For this review, take the finished solid that the model builds, in its own axes (mm). A direction names the side the tool comes from. Coordinates: 2 decimals unless noted, no trailing zeros. Write each loop counter-clockwise with the first axis right and the second up, starting at its lowest first coordinate (ties: lowest second). Pieces come first, ordered by that corner, then holes. Notation, with made-up numbers: (-4.75, 45.25) - (-0.75, 45.25) arc R16 cw to (-0.75, 50.25) - close; hole circle Ø5 at (4.25, -17). An arc over 180 degrees is marked (long way). Use one line per item in the form item = value. Start each with the question number.
1) We need section B-B (x = 0). Give the boundary of the cut face in (y, z), plus the area to 3 significant figures.
2) We need section D-D (y = 5). Count the separate pieces of the cut face and the enclosed holes in it, plus the area to 3 significant figures.
3) We need section A-A (z = 16.5). Give the boundary of the cut face in (x, y).
4) We need section C-C (y = -19.25). Give the boundary of the cut face in (x, z).
5) Mouldability with a two-part tool opening along Z and no side actions: class faces 5 (the flat face through (-12, 0, 1)), 6 (the flat face through (12, 0, 3)), 7 (the cylindrical face through (54.01, 5.09, 25.05)), 8 (the cylindrical face through (24.854, 16.483, 1.986)) as pulls with the +Z half, pulls with the -Z half, needs draft (parallel to the pull), parting line crosses it, or undercut.
6) Tool access review of faces 1 (the flat face through (-13.752, -7.982, 1.986)), 2 (the flat face through (53, 5, 16)), 3 (the cylindrical face through (54.1, 4.86, 1.86)), 4 (the flat face through (-54, -5, 14)): name each direction out of +Z, -Z, +X, -X, +Y, -Y from which nothing blocks a thin tool from reaching the whole face with its end or side.
7) Insertion check: P1, Ø6.5, axis at x = -25.11, y = 14.5, coming from the +Z side; P2, Ø3.5, axis at x = -53, z = 12, coming from the +Y side; P3, Ø1.5, axis at x = -54, z = 18, coming from the -Y side. Each pin has a flat end and moves straight along its axis. Give the tip position at first contact, or say it passes through.
8) For L1, parallel to Y at x = 0, z = 2.2; L2, parallel to X at y = 13, z = 19.25; L3, parallel to Y at x = 53.85, z = 23, list the stretches that pass through material, from the lowest coordinate up. Write a range as from..to.
```python
from build123d import *

# Parameters (mm, degrees)
SKETCH_1_R                  = 33
SKETCH_1_R_2                = 11.05
SKETCH_1_R_3                = 4.05
SKETCH_1_R_4                = 2
EXTRUDE_1_DEPTH             = 3
EXTRUDE_2_DEPTH             = 3
SHEET_METAL_1_OUTLINE_R     = 2
SHEET_METAL_1_OUTLINE_R_2   = 4.05
SHEET_METAL_1_OUTLINE_R_3   = 11.05
SHEET_METAL_1_DEPTH         = 1
SM_EDGE_FLANGE_1_DEPTH      = 20
SM_EDGE_FLANGE_1_BEND_DEPTH = 20
SKETCH_13_R                 = 2.05
CUT_EXTRUDE_1_DEPTH         = 118.974573532


# Read off the part's stored shape, not the designer's step: 转换实体1
# Sheet-metal steps are written as plain solids
with BuildPart() as part:
    # Sketch 1 → 凸台-拉伸1 (new body)
    with BuildSketch(Plane.XY):
        Circle(SKETCH_1_R)
        Circle(SKETCH_1_R_2, mode=Mode.SUBTRACT)
        with Locations((0, -19.25)):
            Circle(SKETCH_1_R_3, mode=Mode.SUBTRACT)
        with Locations((25.11473671, 14.5)):
            Circle(SKETCH_1_R_4, mode=Mode.SUBTRACT)
        with Locations((0, -29)):
            Circle(SKETCH_1_R_4, mode=Mode.SUBTRACT)
        with Locations((-25.11473671, 14.5)):
            Circle(SKETCH_1_R_4, mode=Mode.SUBTRACT)
        with BuildLine():
            Line((-19.57313602, -8.29833395), (-16.97313602, -12.80166605))
            ThreePointArc((-16.97313602, -12.80166605), (-16.487370933, -13.174406711), (-15.880315697, -13.094486373))
            Line((-15.880315697, -13.094486373), (-12.762624243, -11.294486373))
            ThreePointArc((-12.762624243, -11.294486373), (-12.389883582, -10.808721286), (-12.46980392, -10.20166605))
            Line((-12.46980392, -10.20166605), (-15.06980392, -5.69833395))
            ThreePointArc((-15.06980392, -5.69833395), (-15.555569007, -5.325593289), (-16.162624243, -5.405513627))
            Line((-16.162624243, -5.405513627), (-19.280315697, -7.205513627))
            ThreePointArc((-19.280315697, -7.205513627), (-19.653056358, -7.691278714), (-19.57313602, -8.29833395))
        make_face(mode=Mode.SUBTRACT)
    extrude(amount=EXTRUDE_1_DEPTH)

    # 草图3 → 凸台-拉伸2 (add)
    with BuildSketch(Plane.XY):
        with BuildLine():
            ThreePointArc((-18.301945503, -27.459766765), (-32.813072233, 3.507462139), (-12.084283208, 30.707818212))
            Line((-12.084283208, 30.707818212), (-52, 15))
            Line((-52, 15), (-52, -5))
            Line((-52, -5), (-18.301945503, -27.459766765))
        make_face()
        with BuildLine():
            ThreePointArc((18.301945503, -27.459766765), (32.813072233, 3.507462139), (12.084283208, 30.707818212))
            Line((12.084283208, 30.707818212), (52, 15))
            Line((52, 15), (52, -5))
            Line((52, -5), (18.301945503, -27.459766765))
        make_face()
    extrude(amount=EXTRUDE_2_DEPTH)

    # Sheet Metal 1 outline → Sheet Metal 1 (cut)
    with BuildSketch(Plane.XY):
        with BuildLine():
            ThreePointArc((-18.301945503, -27.459766765), (0, -33), (18.301945503, -27.459766765))
            Line((18.301945503, -27.459766765), (52, -5))
            Line((52, -5), (52, 15))
            Line((52, 15), (12.084283208, 30.707818212))
            ThreePointArc((12.084283208, 30.707818212), (0, 33), (-12.084283208, 30.707818212))
            Line((-12.084283208, 30.707818212), (-52, 15))
            Line((-52, 15), (-52, -5))
            Line((-52, -5), (-18.301945503, -27.459766765))
        make_face()
        with BuildLine():
            Line((-16.97313602, -12.80166605), (-19.57313602, -8.29833395))
            ThreePointArc((-19.57313602, -8.29833395), (-19.653056358, -7.691278714), (-19.280315697, -7.205513627))
            Line((-19.280315697, -7.205513627), (-16.162624243, -5.405513627))
            ThreePointArc((-16.162624243, -5.405513627), (-15.555569007, -5.325593289), (-15.06980392, -5.69833395))
            Line((-15.06980392, -5.69833395), (-12.46980392, -10.20166605))
            ThreePointArc((-12.46980392, -10.20166605), (-12.389883582, -10.808721286), (-12.762624243, -11.294486373))
            Line((-12.762624243, -11.294486373), (-15.880315697, -13.094486373))
            ThreePointArc((-15.880315697, -13.094486373), (-16.487370933, -13.174406711), (-16.97313602, -12.80166605))
        make_face(mode=Mode.SUBTRACT)
        with Locations((0, -29)):
            Circle(SHEET_METAL_1_OUTLINE_R, mode=Mode.SUBTRACT)
        with Locations((0, -19.25)):
            Circle(SHEET_METAL_1_OUTLINE_R_2, mode=Mode.SUBTRACT)
        with Locations((-25.11473671, 14.5)):
            Circle(SHEET_METAL_1_OUTLINE_R, mode=Mode.SUBTRACT)
        Circle(SHEET_METAL_1_OUTLINE_R_3, mode=Mode.SUBTRACT)
        with Locations((25.11473671, 14.5)):
            Circle(SHEET_METAL_1_OUTLINE_R, mode=Mode.SUBTRACT)
    extrude(amount=SHEET_METAL_1_DEPTH, mode=Mode.SUBTRACT)

    # 边线-法兰1 section (across the edge) → 边线-法兰1 (add)
    with BuildSketch(Plane(origin=(53, -5, 3), x_dir=(-1, 0, 0), z_dir=(0, 1, 0))):
        with BuildLine():
            Line((-2, 1), (-2, 24))
            Line((-2, 24), (0, 24))
            Line((0, 24), (0, 1))
            ThreePointArc((0, 1), (0.292893219, 0.292893219), (1, 0))
            Line((1, 0), (1, -2))
            ThreePointArc((1, -2), (-1.121320344, -1.121320344), (-2, 1))
        make_face()
    extrude(amount=SM_EDGE_FLANGE_1_DEPTH)

    # 边线-法兰1 section 2 (across the edge) → 边线-法兰1 bend (add)
    with BuildSketch(Plane(origin=(-53, 15, 3), x_dir=(1, 0, 0), z_dir=(0, -1, 0))):
        with BuildLine():
            Line((-2, 1), (-2, 24))
            Line((-2, 24), (0, 24))
            Line((0, 24), (0, 1))
            ThreePointArc((0, 1), (0.292893219, 0.292893219), (1, 0))
            Line((1, 0), (1, -2))
            ThreePointArc((1, -2), (-1.121320344, -1.121320344), (-2, 1))
        make_face()
    extrude(amount=SM_EDGE_FLANGE_1_BEND_DEPTH)

    # 草图13 → 切除-拉伸1 (cut, through all)
    with BuildSketch(Plane(origin=(55, 0, 0), x_dir=(0, 0, -1), z_dir=(1, 0, 0))):
        with Locations((-23, 5)):
            Circle(SKETCH_13_R)
        with Locations((-13, 5)):
            Circle(SKETCH_13_R)
    extrude(amount=-CUT_EXTRUDE_1_DEPTH, mode=Mode.SUBTRACT)


solid = part.part
```
Determined:
q1.outline = (-33, 1) - (-31, 1) - (-31, 3) - (-33, 3) - close; (-27, 1) - (-23.3, 1) - (-23.3, 3) - (-27, 3) - close; (-15.2, 1) - (-11.05, 1) - (-11.05, 3) - (-15.2, 3) - close; (11.05, 1) - (33, 1) - (33, 3) - (11.05, 3) - close
q1.area = 63.6 mm²
q2.separate_pieces = 6
q2.enclosed_holes = 0
q2.area = 240 mm²
q3.outline = (-55, -5) - (-53, -5) - (-53, 15) - (-55, 15) - close; (53, -5) - (55, -5) - (55, 15) - (53, 15) - close
q4.outline = (-30.62, 1) - (-4.05, 1) - (-4.05, 3) - (-30.62, 3) - close; (4.05, 1) - (30.62, 1) - (30.62, 3) - (4.05, 3) - close
q5.face_5 = pulls with the -Z half
q5.face_6 = pulls with the +Z half
q5.face_7 = undercut
q5.face_8 = needs draft
q6.face_1 = +Z, -Z
q6.face_2 = +Z, +Y, -Y
q6.face_3 = -Z, +X, +Y, -Y
q6.face_4 = +Z, -Z, -X, -Y
q7.P1 = 3
q7.P2 = 15
q7.P3 = -5
q8.L1 = -33..-31, -27..-23.3, -15.2..-11.05, 11.05..33
q8.L2 = -55..-53, 53..55
q8.L3 = -5..2.95, 7.05..15
